from build123d import *

# Parameters (mm, degrees)
F1_DEPTH      = 85
F3_W          = 81
F3_H          = 10
F4_DEPTH      = 20
F7_DEPTH      = 13.6
F9_W          = 60
F9_H          = 20
F10_DEPTH     = 2
F12_W         = 20
F12_H         = 60
F13_DEPTH     = 5
F14_T1_DEPTH  = 55
F15_R         = 4.99999
F16_R         = 10
F18_W         = 60
F18_H         = 20
F19_DEPTH     = 4.5
F20_R         = 5
F21_R         = 10.4535447251
F22_W         = 4
F22_H         = 13
F23_DEPTH     = 20
F24_T4_DEPTH  = 107.6390188569
F25_W         = 4
F25_H         = 9.7337032971
F26_DEPTH     = 15
F27_T4_DEPTH  = 81.7292641427
F28_T1_DEPTH  = 4.0324145269
F28_T6_DEPTH  = 55.9380061179
F28_T13_DEPTH = 55.9380061179
F28_T20_DEPTH = 29.9852103224
F28_T26_DEPTH = 55.9380061179


# Not quite as in the source:
# - a fillet or chamfer that OpenCascade refuses, or shapes differently, is made with other operations: its cross-section is extruded or revolved along the edge and cut away or added
# - a fillet or chamfer is up to 0.001 mm smaller than in the source, because OpenCascade refuses the exact size


with BuildPart() as f1:
    # F0 (on Right) → F1 (new body)
    with BuildSketch(Plane.YZ):
        Polygon((-12.1484044939, 63.271041885), (-12.1484044939, -16.728958115), (3.0366472241, -20.0031517962), (3.0366472241, 29.9968482038), (-8.115989967, 29.9968482038), (-8.115989967, 63.271041885), align=None)
    extrude(amount=F1_DEPTH)

    # F3 (on offset) → F4 (cut)
    with BuildSketch(Plane.XY.offset(30.2968482038)):
        with Locations((42.5, -3.115989967)):
            Rectangle(F3_W, F3_H)
    extrude(amount=-F4_DEPTH, mode=Mode.SUBTRACT)

    # F6 (on offset) → F7 (cut)
    with BuildSketch(Plane.XZ.offset(12.1484044939)):
        Polygon((32.5, -16.728958115), (42.5, -16.728958115), (52.5, -16.728958115), (52.5, 13.271041885), (42.5, 13.271041885), (32.5, 13.271041885), align=None)
    extrude(amount=-F7_DEPTH, mode=Mode.SUBTRACT)

    # F9 (on offset) → F10 (cut)
    with BuildSketch(Plane(origin=(0, 3.0366472241, 0), x_dir=(-1, 0, 0), z_dir=(0, 1, 0))):
        with Locations((-42.5, 19.9968482038)):
            Rectangle(F9_W, F9_H)
    extrude(amount=-F10_DEPTH, mode=Mode.SUBTRACT)

    # F12 (on offset) → F13 (join)
    with BuildSketch(Plane(origin=(0, -3.986549235, -18.488813492), x_dir=(1, 0, 0), z_dir=(0, -0.210775525, -0.9775344894))):
        with Locations((75, 38.3494294545)):
            Rectangle(F12_W, F12_H)
        with Locations((10, 38.3494294545)):
            Rectangle(F12_W, F12_H)
    extrude(amount=-F13_DEPTH)

    # F14: fillet of radius 10 on 4 edges, made by hand

    # F14_s2 → F14_t1 (cut)
    with BuildSketch(Plane(origin=(0, -9.2559373608, -42.927175728), x_dir=(1, 0, 0), z_dir=(0, 0.210775525, 0.9775344894))):
        with BuildLine():
            ThreePointArc((75, -68.3494294545), (67.9289321881, -65.4204972664), (65, -58.3494294545))
            Line((65, -58.3494294545), (65, -68.3494294545))
            Line((65, -68.3494294545), (75, -68.3494294545))
        make_face()
        with BuildLine():
            ThreePointArc((10, -68.3494294545), (2.9289321881, -65.4204972664), (0, -58.3494294545))
            Line((0, -58.3494294545), (0, -68.3494294545))
            Line((0, -68.3494294545), (10, -68.3494294545))
        make_face()
        with BuildLine():
            ThreePointArc((20, -58.3494294545), (17.0710678119, -65.4204972664), (10, -68.3494294545))
            Line((10, -68.3494294545), (20, -68.3494294545))
            Line((20, -68.3494294545), (20, -58.3494294545))
        make_face()
        with BuildLine():
            ThreePointArc((75, -68.3494294545), (82.0710678119, -65.4204972664), (85, -58.3494294545))
            Line((85, -58.3494294545), (85, -68.3494294545))
            Line((85, -68.3494294545), (75, -68.3494294545))
        make_face()
    extrude(amount=F14_T1_DEPTH, mode=Mode.SUBTRACT)

    # F15 (radius 5 in the source; OpenCascade refuses exactly that, so slightly less here)
    f15_edges = [f1.edges().sort_by_distance(p)[0] for p in [
        (85, -36.059828, -6.458279),
        (20, -36.059828, -6.458279),
    ]]
    fillet(f15_edges, radius=F15_R)

    # F16
    f16_edges = [f1.edges().sort_by_distance(p)[0] for p in [
        (12.5, 2.036647, 9.996848),
        (72.5, 2.036647, 9.996848),
    ]]
    fillet(f16_edges, radius=F16_R)

    # F18 (on offset) → F19 (cut)
    with BuildSketch(Plane(origin=(0, -8.115989967, 0), x_dir=(-1, 0, 0), z_dir=(0, 1, 0))):
        with Locations((-42.5, 53.271041885)):
            Rectangle(F18_W, F18_H)
    extrude(amount=-F19_DEPTH, mode=Mode.SUBTRACT)

    # F20
    f20_edges = [f1.edges().sort_by_distance(p)[0] for p in [
        (72.5, -10.132197, 63.271042),
        (85, -10.132197, 63.271042),
        (72.5, -10.132197, 43.271042),
        (12.5, -10.132197, 43.271042),
        (12.5, -10.132197, 63.271042),
        (0, -10.132197, 63.271042),
    ]]
    fillet(f20_edges, radius=F20_R)

    # F21
    f21_edges = [f1.edges().sort_by_distance(p)[0] for p in [
        (72.5, 2.460329, 29.996848),
        (12.5, 2.460329, 29.996848),
    ]]
    fillet(f21_edges, radius=F21_R)

    # F22 (on offset) → F23 (join)
    with BuildSketch(Plane(origin=(0, -8.115989967, 0), x_dir=(-1, 0, 0), z_dir=(0, 1, 0))):
        with Locations((-9.9369510557, -6.5)):
            Rectangle(F22_W, F22_H)
    extrude(amount=-F23_DEPTH)

    # F24: chamfer of 20 x 9.3261531631 on 1 edges, made by hand


with BuildPart() as f24_tool2:
    # F24_s3 → F24_t4 (new body)
    with BuildSketch(Plane.YZ.offset(-43.8825583727)):
        Polygon((-8.115989967, 0), (-28.115989967, -9.3261531631), (-28.115989967, 0), align=None)
    extrude(amount=F24_T4_DEPTH)

    split(bisect_by=Plane.XZ.offset(12.1484044939), keep=Keep.TOP)

    split(bisect_by=Plane(origin=(0, -2.9326716098, -13.6011410448), x_dir=(1, 0, 0), z_dir=(0, 0.210775525, 0.9775344894)), keep=Keep.TOP)


with BuildPart() as f1_1:
    add(f1.part)

    # F24_t1: cut F24_tool2
    add(f24_tool2.part, mode=Mode.SUBTRACT)

    # F25 (on face) → F26 (join)
    with BuildSketch(Plane.XZ.offset(12.1484044939)):
        with Locations((75.2541754842, -6.7471974233)):
            Rectangle(F25_W, F25_H)
    extrude(amount=F26_DEPTH)

    # F27: chamfer of 15 x 6.9946148723 on 1 edges, made by hand


with BuildPart() as f27_tool2:
    # F27_s3 → F27_t4 (new body)
    with BuildSketch(Plane.YZ.offset(116.1188075555)):
        Polygon((-12.1484044939, -1.8803457748), (-27.1484044939, -8.8749606471), (-27.1484044939, -1.8803457748), align=None)
    extrude(amount=-F27_T4_DEPTH)

    split(bisect_by=Plane.XZ.offset(12.1484044939), keep=Keep.TOP)

    split(bisect_by=Plane(origin=(0, -2.9326716098, -13.6011410448), x_dir=(1, 0, 0), z_dir=(0, 0.210775525, 0.9775344894)), keep=Keep.TOP)


with BuildPart() as f1_2:
    add(f1_1.part)

    # F27_t1: cut F27_tool2
    add(f27_tool2.part, mode=Mode.SUBTRACT)

    # F28: fillet of radius 10.3811183182 on 2 edges, made by hand

    # F28_s2 → F28_t1 (join)
    with BuildSketch(Plane.XZ.offset(8.115989967)):
        with BuildLine():
            ThreePointArc((42.8811183182, 13.271041885), (35.5405591591, 10.2304827259), (32.5, 2.8899235668))
            Line((32.5, 2.8899235668), (32.5, 13.271041885))
            Line((32.5, 13.271041885), (42.8811183182, 13.271041885))
        make_face()
        with BuildLine():
            ThreePointArc((52.5, 2.8899235668), (49.4594408409, 10.2304827259), (42.1188816818, 13.271041885))
            Line((42.1188816818, 13.271041885), (52.5, 13.271041885))
            Line((52.5, 13.271041885), (52.5, 2.8899235668))
        make_face()
    extrude(amount=F28_T1_DEPTH)


with BuildPart() as f28_tool4:
    # F28_s5 → F28_t6 (new body)
    with BuildSketch(Plane.XZ.offset(38.1012002894)):
        with BuildLine():
            ThreePointArc((42.8811183182, 13.271041885), (35.5405591591, 10.2304827259), (32.5, 2.8899235668))
            Line((32.5, 2.8899235668), (32.5, 13.271041885))
            Line((32.5, 13.271041885), (42.8811183182, 13.271041885))
        make_face()
    extrude(amount=-F28_T6_DEPTH)

    split(bisect_by=Plane.XZ.offset(-1.0366472241), keep=Keep.TOP)

    split(bisect_by=Plane.XY.offset(10.2968482038), keep=Keep.BOTTOM)

    split(bisect_by=Plane.XZ.offset(8.115989967), keep=Keep.BOTTOM)


with BuildPart() as f1_3:
    add(f1_2.part)

    # F28_t3: union F28_tool4
    add(f28_tool4.part)


with BuildPart() as f28_tool11:
    # F28_s12 → F28_t13 (new body)
    with BuildSketch(Plane.XZ.offset(38.1012002894)):
        with BuildLine():
            ThreePointArc((42.8811183182, 13.271041885), (35.5405591591, 10.2304827259), (32.5, 2.8899235668))
            Line((32.5, 2.8899235668), (32.5, 13.271041885))
            Line((32.5, 13.271041885), (42.8811183182, 13.271041885))
        make_face()
    extrude(amount=-F28_T13_DEPTH)

    split(bisect_by=Plane.XY.offset(9.9968482038), keep=Keep.BOTTOM)

    split(bisect_by=Plane.XZ.offset(8.115989967), keep=Keep.BOTTOM)

    split(bisect_by=Plane.XZ.offset(-3.0366472241), keep=Keep.TOP)


with BuildPart() as f1_4:
    add(f1_3.part)

    # F28_t10: union F28_tool11
    add(f28_tool11.part)


with BuildPart() as f28_tool18:
    # F28_s19 → F28_t20 (new body)
    with BuildSketch(Plane.XZ.offset(12.1484044939)):
        with BuildLine():
            ThreePointArc((52.5, 2.8899235668), (49.4594408409, 10.2304827259), (42.1188816818, 13.271041885))
            Line((42.1188816818, 13.271041885), (52.5, 13.271041885))
            Line((52.5, 13.271041885), (52.5, 2.8899235668))
        make_face()
    extrude(amount=-F28_T20_DEPTH)

    split(bisect_by=Plane.XY.offset(10.2968482038), keep=Keep.BOTTOM)

    split(bisect_by=Plane.XZ.offset(-1.0366472241), keep=Keep.TOP)


with BuildPart() as f1_5:
    add(f1_4.part)

    # F28_t17: union F28_tool18
    add(f28_tool18.part)


with BuildPart() as f28_tool24:
    # F28_s25 → F28_t26 (new body)
    with BuildSketch(Plane.XZ.offset(38.1012002894)):
        with BuildLine():
            ThreePointArc((52.5, 2.8899235668), (49.4594408409, 10.2304827259), (42.1188816818, 13.271041885))
            Line((42.1188816818, 13.271041885), (52.5, 13.271041885))
            Line((52.5, 13.271041885), (52.5, 2.8899235668))
        make_face()
    extrude(amount=-F28_T26_DEPTH)

    split(bisect_by=Plane.XY.offset(9.9968482038), keep=Keep.BOTTOM)

    split(bisect_by=Plane.XZ.offset(8.115989967), keep=Keep.BOTTOM)

    split(bisect_by=Plane.XZ.offset(-3.0366472241), keep=Keep.TOP)


with BuildPart() as f1_6:
    add(f1_5.part)

    # F28_t23: union F28_tool24
    add(f28_tool24.part)


solid = f1_6.part
Verification items for the finished model (mm, model axes). A direction names the side the tool comes from. Give positions to 0.01 mm unless a question says otherwise; leave off trailing zeros. Loops run counter-clockwise (first coordinate to the right, second up) from the corner with the lowest first, then second, coordinate; pieces in that order, holes last. Notation, with made-up numbers: (-38.5, -3) - (-33.5, -3) arc R15 cw to (-33.5, 8) - close; hole circle Ø4 at (57.25, 64.25). An arc over 180 degrees is marked (long way). Write item = value, one per line. Start each with the question number.
Q1. Cross-section at B-B, the plane z = 47. Enter the section's corners in (x, y), and give its area (3 significant figures).
Q2. Mould release check, pull along X, two halves, no side actions. Record for faces 1 (the face through (7.937, -18, -7)), 2 (the face through (52.5, -5, -7)), 3 (the face through (83.574, -36.192, -7.968)): released by +X, released by -X, zero draft, split by the parting line, or undercut.
Q3. Tool access check on faces 4 (the face through (34.356, -6.955, 8.814)), 5 (the face through (10.996, -10.16, 61.845)), 6 (the face through (15.431, 2.467, 12.924)), 7 (the face through (18.496, -36.176, -7.892)), 8 (the face through (9.909, -19.185, -5.162)). Record the directions out of +Z, -Z, +X, -X, +Y, -Y that give a thin tool (end or side, any length) a straight path to the whole face; none if there is none.
Q4. Thickness scan on line 1 (X direction, y = -10, z = -8.5); line 2 (Y direction, x = 33, z = 39.5); line 3 (X direction, y = -7, z = 14). Record the ranges inside material, lowest first.
Q5. Cross-section at D-D, the plane x = 40.5. Enter the section's corners in (y, z), and give its area (3 significant figures).
Q6. Depth check by flat-ended pin: P1, Ø20, axis at x = 8, z = 22.5, coming from the -Y side; P2, Ø11.5, axis at y = -42.5, z = -13, coming from the +X side; P3, Ø1.6, axis at x = 84, y = -4, coming from the +Z side; P4, Ø2, axis at x = 63.5, y = -19.5, coming from the +Z side. Enter the tip coordinate at first touch or a pass-through.
Q7. Cross-section at C-C, the plane y = -9.5. Enter the section's corners in (x, z).
Q8. Cross-section at A-A, the plane x = 61. Enter the section's corners in (y, z), and give its area (3 significant figures).
Answer key:
q1.outline = (0, -12.15) - (12.66, -12.15) - (12.66, -8.12) - (0, -8.12) - close; (72.34, -12.15) - (85, -12.15) - (85, -8.12) - (72.34, -8.12) - close
q1.area = 102 mm^2
q2.face_1 = released by -X
q2.face_2 = undercut
q2.face_3 = released by +X
q3.face_4 = -Y
q3.face_5 = +Z, +Y, -Y
q3.face_6 = +Z, +Y
q3.face_7 = +Z
q3.face_8 = +Z, +X, -X
q4.line_1 = 0 to 32.5, 52.5 to 85
q4.line_2 = -12.15 to -8.12
q4.line_3 = 0 to 2, 83 to 85
q5.outline = (-12.15, -16.73) - (3.04, -20) - (3.04, 10) - (1.45, 10) - (1.45, -16.73) - close; (-12.15, 12.99) - (-8.12, 12.99) - (-8.12, 43.27) - (-12.15, 43.27) - close
q5.area = 189 mm^2
q6.P1 = -12.15
q6.P2 = 85
q6.P3 = 30
q6.P4 = through
q7.outline = (0, -17.3) - (85, -17.3) - (85, 58.27) arc R5 ccw to (80, 63.27) - (77.5, 63.27) arc R5 ccw to (72.5, 58.27) - (72.5, 48.27) arc R5 cw to (67.5, 43.27) - (17.5, 43.27) arc R5 cw to (12.5, 48.27) - (12.5, 58.27) arc R5 ccw to (7.5, 63.27) - (5, 63.27) arc R5 ccw to (0, 58.27) - close; hole (32.5, -16.73) - (52.5, -16.73) - (52.5, 2.89) arc R10.38 ccw to (42.5, 13.26) arc R10.38 ccw to (32.5, 2.89) - close
q8.outline = (-12.15, -16.73) - (3.04, -20) - (3.04, 10) - (1.04, 10) - (1.04, 10.3) - (-8.12, 10.3) - (-8.12, 43.27) - (-12.15, 43.27) - close
q8.area = 568 mm^2
